Drawing for the job (mm, zero at the part's lowest x, y, z). Give positions to 0.01 mm unless a question says otherwise; leave off trailing zeros. Order: outer loops, then holes, each group sorted by start corner. A loop starts at its lowest first (then second) coordinate and runs counter-clockwise, first axis right, second up. Notation, with made-up numbers: M 82,-33.5 L 95,-33.5 A18 ccw 95,-14.5 Z; hole C -30.5,46.25 d9. An arc over 180 degrees is marked long. Answer as a JSON object with one key per item and string values.
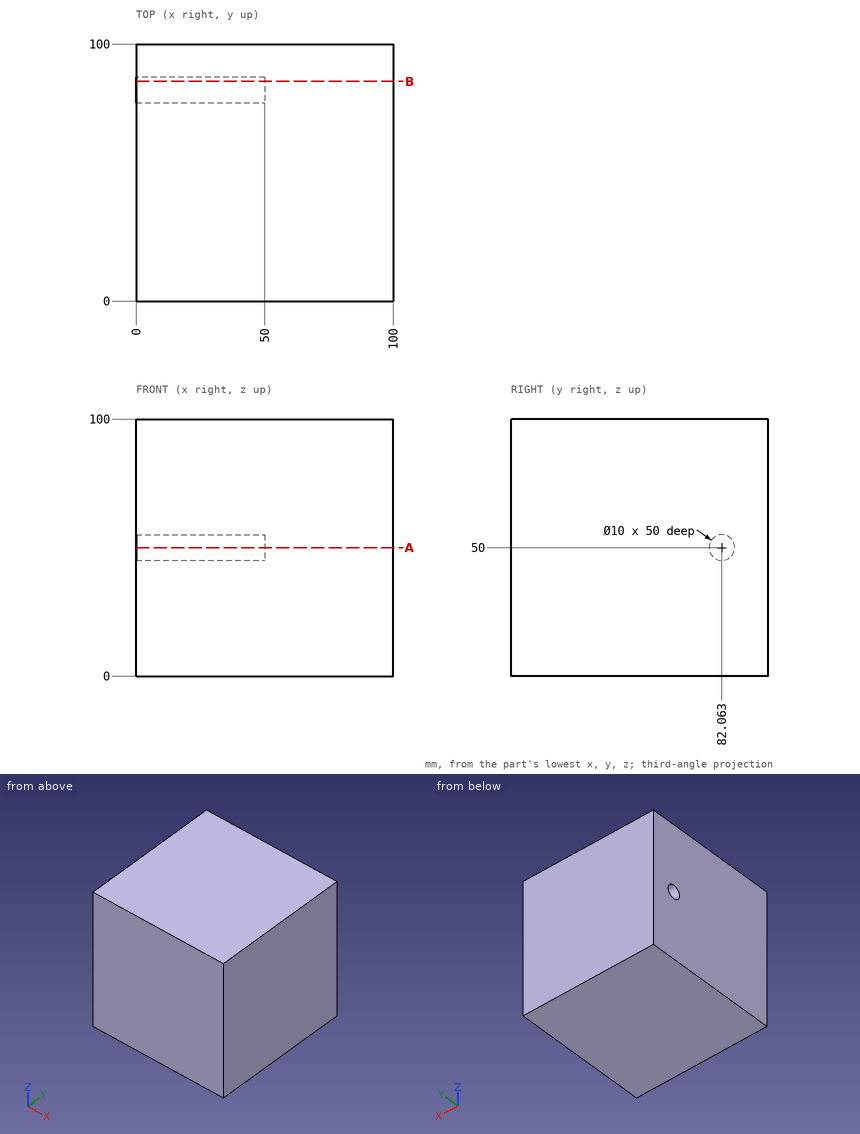
1. Pin check, flat tip, straight feed: P1, Ø6, axis at y = 82.06, z = 50, coming from the -X side. Stop position of the tip, or through.
Worked answers:
{"P1": "stops at x = 50"}
2. Cut at B-B on y = 85.5. Give the cut face in (x, z).
Worked answers:
{"outline": "M 0,0 L 100,0 L 100,100 L 0,100 L 0,53.63 L 50,53.63 L 50,46.37 L 0,46.37 Z"}
3. Probe line 1 along Z through (x, y) = (34, 80.5); line 2 along Y through (x, z) = (17.5, 47); line 3 along Z through (x, y) = (25.5, 86). List the from-to ranges inside material, lowest first.
Worked answers:
{"line 1": "z = 0 to 45.25, 54.75 to 100", "line 2": "y = 0 to 78.06, 86.06 to 100", "line 3": "z = 0 to 46.92, 53.08 to 100"}
4. Cut at A-A on z = 50. Give the cut face in (x, y).
Worked answers:
{"outline": "M 0,0 L 100,0 L 100,100 L 0,100 L 0,87.06 L 50,87.06 L 50,77.06 L 0,77.06 Z"}
